```python
from build123d import *

# Parameters (mm, degrees)
SKETCH_1_R          = 12.5
EXTRUDE_1_DEPTH     = 356
SKETCH_2_R          = 10
CUT_EXTRUDE_1_DEPTH = 20
SKETCH_3_R          = 3
CUT_EXTRUDE_2_DEPTH = 800
SKETCH_4_R          = 12
CUT_EXTRUDE_3_DEPTH = 20


with BuildPart() as part:
    # 草图1 → 凸台-拉伸1 (new body, symmetric)
    with BuildSketch(Plane(origin=(0, 0, 0), x_dir=(1, 0, 0), z_dir=(0, 1, 0))):
        Circle(SKETCH_1_R)
    extrude(amount=EXTRUDE_1_DEPTH, both=True)

    # 草图2 → 切除-拉伸1 (cut)
    with BuildSketch(Plane(origin=(0, 356, 0), x_dir=(1, 0, 0), z_dir=(0, 1, 0))):
        Circle(SKETCH_2_R)
    extrude(amount=-CUT_EXTRUDE_1_DEPTH, mode=Mode.SUBTRACT)

    # 草图3 → 切除-拉伸2 (cut)
    with BuildSketch(Plane(origin=(0, 356, 0), x_dir=(1, 0, 0), z_dir=(0, 1, 0))):
        Circle(SKETCH_3_R)
    extrude(amount=-CUT_EXTRUDE_2_DEPTH, mode=Mode.SUBTRACT)

    # 草图4 → 切除-拉伸3 (cut)
    with BuildSketch(Plane.XZ.offset(356)):
        Circle(SKETCH_4_R)
    extrude(amount=-CUT_EXTRUDE_3_DEPTH, mode=Mode.SUBTRACT)


solid = part.part
```
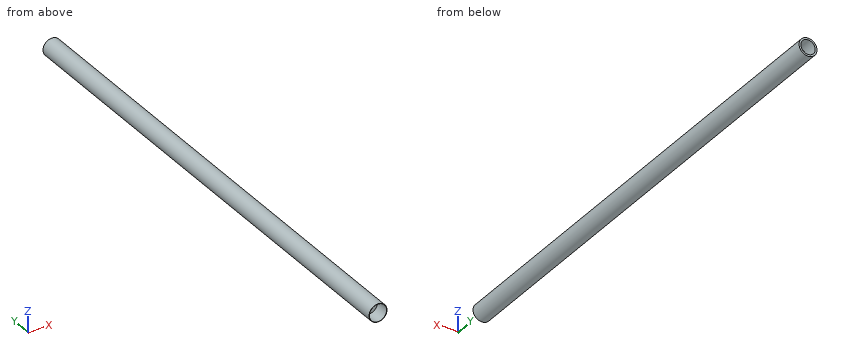
Geometry check sheet. Reference: the model listing, model coordinates, mm. Round coordinates to 2 decimals unless told otherwise and drop trailing zeros. Loops run counter-clockwise (first coordinate to the right, second up) from the corner with the lowest first, then second, coordinate; pieces in that order, holes last. Notation, with made-up numbers: (19.5, -29) - (70.5, -29) arc R10 ccw to (70.5, -15) - close; hole circle Ø6 at (-12.5, -6). An arc over 180 degrees is marked (long way). Use a Markdown table: item, result.
Q1. Go/stop test with flat-tipped pins: P1, Ø4, axis at x = 1, z = -5, coming from the +Y side; P2, Ø8, axis at y = -66.5, z = -9, coming from the +X side; P3, Ø4, axis at x = 7, z = -5, coming from the -Y side. Record where each tip stops, or that it passes through.
Solutions:
| item | result |
|---|---|
| P1 | stops at y = 336 |
| P2 | stops at x = 11.46 |
| P3 | stops at y = -336 |
Q2. Cross-section at A-A on y = 137. Record the cut outline in (x, z), plus the area to 3 significant figures.
Solutions:
| item | result |
|---|---|
| outline | circle Ø25 at (0, 0); hole circle Ø6 at (0, 0) |
| area | 463 mm2 |
Q3. Material ranges on line 1 (X direction, y = -126.5, z = 0); line 2 (Z direction, x = 0, y = 351.5), recorded low to high.
Solutions:
| item | result |
|---|---|
| line 1 | x = -12.5 to -3, 3 to 12.5 |
| line 2 | z = -12.5 to -10, 10 to 12.5 |
